Autodesk Inventor part; units mm, degrees
ref_plane "YZ Plane" through (0, 0, 0) normal (1, 0, 0) x (0, 1, 0)
ref_plane "XZ Plane" through (0, 0, 0) normal (0, 1, 0) x (-1, 0, 0)
ref_plane "XY Plane" through (0, 0, 0) normal (0, 0, 1) x (1, 0, 0)
sketch "Esquisse9" plane through (0, 0, 0) normal (0, 1, 0) x (-1, 0, 0)
  line L0 (0, 0) -> (100, 0)
  line L1 (120, 0) -> (-20, 0) construction
  dimension "d20" = 100
sketch "Esquisse10" plane through (0, 0, 0) normal (1, 0, 0) x (0, 1, 0)
  circle A0 centre (0, 0) radius 30
  circle A1 centre (0, 0) radius 23
  dimension "d22" = 60
  dimension "d23" = 46
sweep "Balayage2" add profiles "Esquisse10" path "Esquisse9"
sketch "Esquisse11" plane through (0, 0, 0) normal (1, 0, 0) x (0, 0, -1)
  circle A0 centre (0, 0) radius 23 construction
  circle A1 centre (0, 0) radius 30 construction
  circle A2 centre (0, 0) radius 23
  circle A3 centre (0, 0) radius 25
  dimension "d26" = 50
extrude "Extrusion4" add sketch "Esquisse11" along normal blind 10
sketch "Esquisse15" plane through (-100, 0, 0) normal (-1, 0, 0) x (0, 0, 1)
  circle A0 centre (0, 0) radius 23
  circle A1 centre (0, 0) radius 25
  dimension "d41" = 46
  dimension "d42" = 50
extrude "Extrusion6" cut sketch "Esquisse15" against normal blind 10
properties part number "P008_CanonBout"
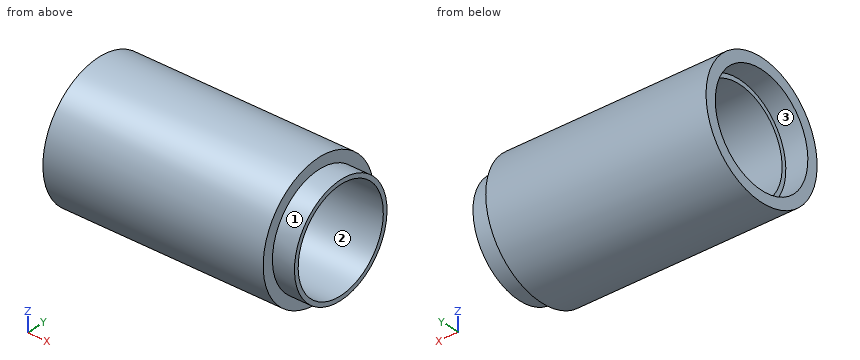
Model file for the job. Use its own axes, mm. Face numbers are marked on the shaded views. A direction names the side the tool comes from. Give positions to 0.01 mm unless a question says otherwise; leave off trailing zeros. Write each loop counter-clockwise with the first axis right and the second up, starting at its lowest first coordinate (ties: lowest second). Pieces come first, ordered by that corner, then holes. Notation, with made-up numbers: (60, 10.5) -> (117, 10.5) arc R17 ccw to (117, 19.5) -> close; hole circle Ø11 at (35, 19.25). An arc over 180 degrees is marked (long way). Write item = value, one per line.
(1) Slice it at B-B, the plane y = -18. Give the cut face in (x, z).
Determined:
outline = (-100, -24) -> (0, -24) -> (0, -17.35) -> (10, -17.35) -> (10, -14.32) -> (-90, -14.32) -> (-90, -17.35) -> (-100, -17.35) -> close; (-100, 17.35) -> (-90, 17.35) -> (-90, 14.32) -> (10, 14.32) -> (10, 17.35) -> (0, 17.35) -> (0, 24) -> (-100, 24) -> close
(2) Probe line 1 along Y through (x, z) = (-22.5, 0); line 2 along Z through (x, y) = (-0.5, 0.5); line 3 along X through (y, z) = (-23.5, -4). List the from-to ranges inside material, lowest first.
Determined:
line_1 = -30 to -23, 23 to 30
line_2 = -30 to -22.99, 22.99 to 30
line_3 = -90 to 10
(3) Flat gauge pins, fed straight in: P1, Ø3, axis at x = -83.5, y = 1.5, coming from the -Z side; P2, Ø6, axis at x = -65.5, y = 13.5, coming from the -Z side; P3, Ø4, axis at x = -9.5, z = 16, coming from the +Y side; P4, Ø25, axis at y = -3, z = -4.5, coming from the -X side. Where does each tip first touch, or does it go through?
Determined:
P1 = -30
P2 = -28.1
P3 = 26.53
P4 = through
(4) Slice it at C-C, the plane x = -10.5. Give the cut face in (y, z), then the cut area to 3 significant figures.
Determined:
outline = circle Ø60 at (0, 0); hole circle Ø46 at (0, 0)
area = 1,170 mm2
(5) Tool access for the marked faces 1, 2 and 3: list every direction of +Z, -Z, +X, -X, +Y, -Y with a clear straight run to the whole face (end or side of a thin tool).
Determined:
face_1 = +X
face_2 = +X, -X
face_3 = -X
(6) Slice it at A-A, the plane z = 13.5. Give the cut face in (x, y), then the cut area to 3 significant figures.
Determined:
outline = (-100, -26.79) -> (0, -26.79) -> (0, -21.04) -> (10, -21.04) -> (10, -18.62) -> (-90, -18.62) -> (-90, -21.04) -> (-100, -21.04) -> close; (-100, 21.04) -> (-90, 21.04) -> (-90, 18.62) -> (10, 18.62) -> (10, 21.04) -> (0, 21.04) -> (0, 26.79) -> (-100, 26.79) -> close
area = 1,630 mm2
